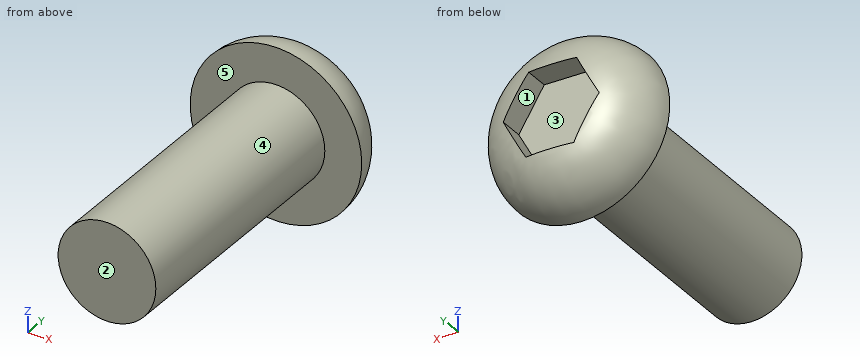
from build123d import *

# Parameters (mm, degrees)
F0_R     = 4.191
F1_DEPTH = 2.5654
F2_R     = 2.3876
F3_DEPTH = 12.7
F5_DEPTH = 1.27


# Not quite as in the source:
# - a fillet or chamfer that OpenCascade refuses, or shapes differently, is made with other operations: its cross-section is extruded or revolved along the edge and cut away or added


with BuildPart() as f1:
    # F0 (on Front) → F1 (new body)
    with BuildSketch(Plane.XZ):
        Circle(F0_R)
    extrude(amount=-F1_DEPTH)

    # F2 (on face) → F3 (join)
    with BuildSketch(Plane.XZ):
        Circle(F2_R)
    extrude(amount=F3_DEPTH)

    # F4 (on face) → F5 (cut)
    with BuildSketch(Plane(origin=(0, 2.5654, 0), x_dir=(-1, 0, 0), z_dir=(0, 1, 0))):
        Polygon((-2.3449476001, 0.0811547043), (-1.2427558356, -1.9902068401), (1.1021917645, -2.0713615444), (2.3449476001, -0.0811547043), (1.2427558356, 1.9902068401), (-1.1021917645, 2.0713615444), align=None)
    extrude(amount=-F5_DEPTH, mode=Mode.SUBTRACT)

    # F6: fillet of radius 2.5654 on 1 edges, made by hand

    # F6_s1 → F6_t2 (revolve, cut)
    with BuildSketch(Plane.XY):
        with BuildLine():
            ThreePointArc((4.191, 0), (3.4396117365, 1.8140117365), (1.6256, 2.5654))
            Line((1.6256, 2.5654), (4.191, 2.5654))
            Line((4.191, 2.5654), (4.191, 0))
        make_face()
    revolve(axis=Axis((0, 2.5654, 0), (0, -1, 0)), mode=Mode.SUBTRACT)


solid = f1.part
Can you work these out from the model? Positions are in its coordinate system, mm. Face numbers are marked on the shaded views. A direction names the side the tool comes from. Round coordinates to 2 decimals unless told otherwise and drop trailing zeros. Order: outer loops, then holes, each group sorted by start corner. A loop starts at its lowest first (then second) coordinate and runs counter-clockwise, first axis right, second up. Notation, with made-up numbers: (30, 4) -> (79, 4) arc R27 ccw to (79, 25) -> close; hole circle Ø11 at (-34, 22.25). An arc over 180 degrees is marked (long way). Write each question's results on one line, items separated by ' | '. Start each with the question number.
Item 1: Thinking about a two-plate mould opening in Z: for the marked faces 3, 4 and 5, which applies, +Z half, -Z half, draft (parallel to the pull), parting line (faces both ways), or undercut?
Item 2: Please list where these lines run through material, in increasing order: L1, parallel to Y at x = 0.5, z = -1; L2, parallel to Z at x = -2, y = -11.5; L3, parallel to Y at x = 1.5, z = -2.
Item 3: Which directions (+Z, -Z, +X, -X, +Y, -Y) give clear straight access to the entire face, cutting with the end or side of a thin tool? Please do the marked faces 1 and 2.
Item 4: If we section it at A-A, the plane y = -6: Write out the boundary of the cut face in (x, z), then the cut area to 3 significant figures.
Item 5: Will these pins go through, and if not, where does the flat tip stop? pin 1 (4 mm diameter, centred on y = -6.5, z = -3, fed in from +X); pin 2 (5 mm diameter, centred on x = -2, y = -6, fed in from +Z); pin 3 (4.5 mm diameter, centred on x = -1, z = -0.5, fed in from +Y); pin 4 (1 mm diameter, centred on x = -1.5, y = -10.5, fed in from -Z).
Results:
1) face 3: undercut | face 4: parting line | face 5: draft
2) L1: y = -12.7 to 1.3 | L2: z = -1.3 to 1.3 | L3: y = 0 to 2.41
3) face 1: +Y | face 2: +Z, -Z, +X, -X, -Y
4) outline: circle Ø4.78 at (0, 0) | area: 17.9 mm2
5) pin 1: stops at x = 2.17 | pin 2: stops at z = 2.39 | pin 3: stops at y = 2.53 | pin 4: stops at z = -2.17
